```python
from build123d import *

# Parameters (mm, degrees)
SKETCH1_R           = 13.5
BOSS_EXTRUDE1_DEPTH = 3.5
CUT_EXTRUDE1_REACH  = 21.41
CIRPATTERN1_COUNT   = 5
CUT_EXTRUDE2_REACH  = 21.41
SKETCH3_W           = 1.767766952
SKETCH3_H           = 1.767766952


with BuildPart() as part:
    # Sketch1 → Boss-Extrude1 (new body)
    with BuildSketch(Plane(origin=(0, 0, 0), x_dir=(0, 0, -1), z_dir=(1, 0, 0))):
        Circle(SKETCH1_R)
    extrude(amount=BOSS_EXTRUDE1_DEPTH)

    # Sketch2 → Cut-Extrude1 (cut, up to next)
    with BuildSketch(Plane(origin=(0, 0, 0), x_dir=(0, 0, -1), z_dir=(1, 0, 0)), mode=Mode.PRIVATE) as cut_extrude1_sk1:
        with BuildLine():
            ThreePointArc((0, 5.335224169), (-2.256377168, 7.208861271), (-3.687303072, 9.768979428))
            ThreePointArc((-3.687303072, 9.768979428), (-2.000654027, 11.080188439), (0, 11.829479796))
            ThreePointArc((0, 11.829479796), (2.000654027, 11.080188439), (3.687303072, 9.768979428))
            ThreePointArc((3.687303072, 9.768979428), (2.256377168, 7.208861271), (0, 5.335224169))
        make_face()
    cut_extrude1_tool1 = extrude(cut_extrude1_sk1.sketch, amount=CUT_EXTRUDE1_REACH, mode=Mode.PRIVATE) & part.part
    cut_extrude1 = cut_extrude1_tool1.solids().sort_by_distance((0, 8.878443, 0))[0]
    add(cut_extrude1, mode=Mode.SUBTRACT)

    # CirPattern1: Cut-Extrude1 ×5 about axis
    cirpattern1_axis = Axis((0, 0, 0), (1, 0, 0))
    for i in range(1, CIRPATTERN1_COUNT):
        add(cut_extrude1.rotate(cirpattern1_axis, i * 360 / CIRPATTERN1_COUNT), mode=Mode.SUBTRACT)

    # Sketch3 → Cut-Extrude2 (cut, up to next)
    with BuildSketch(Plane(origin=(0, 0, 0), x_dir=(0, 0, -1), z_dir=(1, 0, 0)), mode=Mode.PRIVATE) as cut_extrude2_sk1:
        Rectangle(SKETCH3_W, SKETCH3_H)
    cut_extrude2_tool1 = extrude(cut_extrude2_sk1.sketch, amount=CUT_EXTRUDE2_REACH, mode=Mode.PRIVATE) & part.part
    add(cut_extrude2_tool1.solids().sort_by_distance((0, 0, 0))[0], mode=Mode.SUBTRACT)


solid = part.part
```
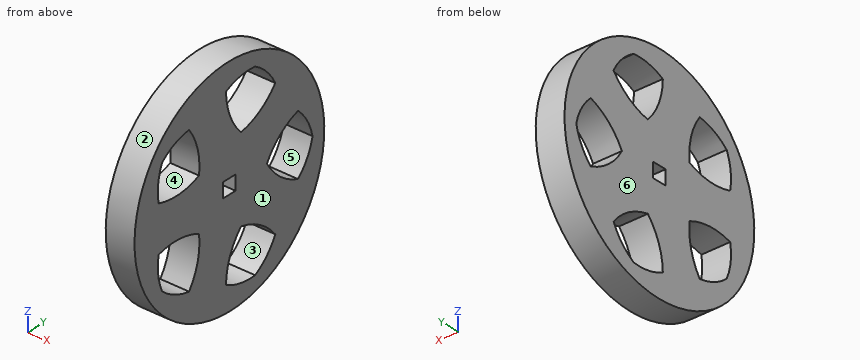
For this review, take the finished solid that the model builds, in its own axes (mm). Face numbers are marked on the shaded views. A direction names the side the tool comes from. Round coordinates to 2 decimals unless told otherwise and drop trailing zeros. Write each loop counter-clockwise with the first axis right and the second up, starting at its lowest first coordinate (ties: lowest second). Pieces come first, ordered by that corner, then holes. Notation, with made-up numbers: (3.5, -29.5) - (33.5, -29.5) arc R15 ccw to (33.5, -10.5) - close; hole circle Ø5 at (-32.75, -3). An arc over 180 degrees is marked (long way). Answer as a JSON object with one key per item and string values.
1. We need section B-B on z = 9.75. Give the boundary of the cut face in (x, y), then the cut area to 3 significant figures.
Response values:
{"outline": "(0, -9.34) - (3.5, -9.34) - (3.5, -0.45) - (0, -0.45) - close; (0, 5.48) - (3.5, 5.48) - (3.5, 9.34) - (0, 9.34) - close", "area": "44.6 mm2"}
2. Tool access review of the marked faces 5 and 6: name each direction out of +Z, -Z, +X, -X, +Y, -Y from which nothing blocks a thin tool from reaching the whole face with its end or side.
Response values:
{"face 5": "+X, -X", "face 6": "+Z, -Z, -X, +Y, -Y"}
3. We need section C-C on y = -8.5. Give the boundary of the cut face in (x, z), then the cut area to 3 significant figures.
Response values:
{"outline": "(0, -10.49) - (3.5, -10.49) - (3.5, -7.75) - (0, -7.75) - close; (0, -2.44) - (3.5, -2.44) - (3.5, 2.44) - (0, 2.44) - close; (0, 7.75) - (3.5, 7.75) - (3.5, 10.49) - (0, 10.49) - close", "area": "36.2 mm2"}
4. We need section D-D on y = 0. Give the boundary of the cut face in (x, z), then the cut area to 3 significant figures.
Response values:
{"outline": "(0, -13.5) - (3.5, -13.5) - (3.5, -10.67) - (0, -10.67) - close; (0, -7.77) - (3.5, -7.77) - (3.5, -0.88) - (0, -0.88) - close; (0, 0.88) - (3.5, 0.88) - (3.5, 7.77) - (0, 7.77) - close; (0, 10.67) - (3.5, 10.67) - (3.5, 13.5) - (0, 13.5) - close", "area": "68.0 mm2"}
5. Draft analysis for pull direction Y (two halves, no side actions). For the marked faces 1, 2, 3 and 4, state which applies: +Y half, -Y half, draft (parallel to the pull), parting line (faces both ways), or undercut.
Response values:
{"face 1": "draft", "face 2": "parting line", "face 3": "undercut", "face 4": "undercut"}
6. To check wall thickness, follow line 1 along Y through (x, z) = (3.2, -5.5); line 2 along Z through (x, y) = (0.5, -5.25); line 3 along Z through (x, y) = (2.95, 3.5). State the ranges of each line that lie inside material, in increasing order.
Response values:
{"line 1": "y = -12.33 to -10.04, -4.38 to 1.28, 3.08 to 12.33", "line 2": "z = -12.44 to -7.95, -2.77 to 2.77, 7.95 to 12.44", "line 3": "z = -13.04 to -11.27, -5.68 to 5.68, 11.27 to 13.04"}
7. We need section A-A on x = 0.65. Give the boundary of the cut face in (y, z), then the cut area to 3 significant figures.
Response values:
{"outline": "circle Ø27 at (0, 0); hole (-10.07, -2.76) arc R7.09 ccw to (-9.57, -6.95) arc R7.09 ccw to (-5.74, -8.73) arc R8.01 ccw to (-4.32, -3.14) arc R8.01 ccw to start; hole (-10.07, 2.76) arc R8.01 ccw to (-4.32, 3.14) arc R8.01 ccw to (-5.74, 8.73) arc R7.09 ccw to (-9.57, 6.95) arc R7.09 ccw to start; hole (-0.88, -0.88) - (0.88, -0.88) - (0.88, 0.88) - (-0.88, 0.88) - close; hole (-0.49, -10.43) arc R7.09 ccw to (3.66, -11.25) arc R7.09 ccw to (6.53, -8.15) arc R8.01 ccw to (1.65, -5.07) arc R8.01 ccw to start; hole (-0.49, 10.43) arc R8.01 ccw to (1.65, 5.07) arc R8.01 ccw to (6.53, 8.15) arc R7.09 ccw to (3.66, 11.25) arc R7.09 ccw to start; hole (5.34, 0) arc R8.01 ccw to (9.77, -3.69) arc R7.09 ccw to (11.83, 0) arc R7.09 ccw to (9.77, 3.69) arc R8.01 ccw to start", "area": "420 mm2"}
8. For pin 1 Ø0.5 at (x, z) = (1, -0.5) entering from -Y, flat-tipped, find the tip position at first contact; note if it passes through.
Response values:
{"pin 1": "stops at y = -13.5"}
